The model under review builds one solid part; all positions refer to its coordinate system, in mm. Face numbers are marked on the shaded views. A direction names the side the tool comes from. Coordinates: 2 decimals unless noted, no trailing zeros. Write each loop counter-clockwise with the first axis right and the second up, starting at its lowest first coordinate (ties: lowest second). Pieces come first, ordered by that corner, then holes. Notation, with made-up numbers: (-15.75, 17) - (38.25, 17) arc R30 cw to (38.25, 51) - close; hole circle Ø7 at (50.5, 28.25). An arc over 180 degrees is marked (long way). Return JSON: item names as keys, results as strings. Group by question number.
(1) We need section A-A on z = -1. Give the number of separate pieces and of enclosed holes in the cut face, then the cut area to 3 significant figures.
(2) We need section C-C on z = 7. State the section outline as (x, y) points, then the cut area to 3 significant figures.
(3) Draft analysis for pull direction Y (two halves, no side actions). For the marked faces 1, 2, 3 and 4, state which applies: released by +Y, released by -Y, zero draft, split by the parting line, or undercut.
(4) To check wall thickness, follow L1, parallel to X at y = -2.75, z = 7; L2, parallel to Z at x = 0, y = -2.5; L3, parallel to Z at x = 0, y = -2. State the ranges of each line that lie inside material, in increasing order. Write a range as from..to.
(5) We need section B-B on x = 0. State the section outline as (y, z) points.
(6) We need section D-D on y = 0.5. State the section outline as (x, z) points.
(7) Tool access review of the marked faces 5, 6, 7 and 8: name each direction out of +Z, -Z, +X, -X, +Y, -Y from which nothing blocks a thin tool from reaching the whole face with its end or side.
(8) For pin 1 Ø0.9 at (x, z) = (4.5, -1) entering from +Y; pin 2 Ø3.5 at (x, y) = (-1.5, 4) entering from +Z; pin 3 Ø0.9 at (y, z) = (-4.5, -0.5) entering from -X, all flat-tipped, find the tip position at first contact; note any pin that passes through.
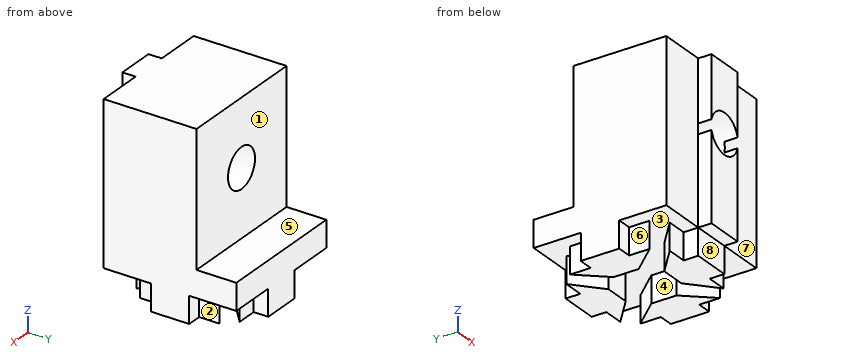
```python
from build123d import *

# Parameters (mm, degrees)
SKETCH1_W                         = 10
SKETCH1_H                         = 10
MAIN_DEPTH                        = 12
ANTIROTATIONSYSTEM_DEPTH          = 2
CIRPATTERN1_COUNT                 = 4
SKETCH3_W                         = 10
SKETCH3_H                         = 10
MAKERBEAMSQUAREHOLEFORSCREW_DEPTH = 3
SKETCH5_W                         = 2.9
SKETCH5_H                         = 12
MAKERBEAMRAIL_DEPTH               = 1
SKETCH4_R                         = 1.5
VERTICALMAKERBEAMHOLE_DEPTH       = 9


with BuildPart() as part:
    # Sketch1 → Main (new body)
    with BuildSketch(Plane.XY):
        Rectangle(SKETCH1_W, SKETCH1_H)
    extrude(amount=MAIN_DEPTH)

    # Sketch2 → AntiRotationSystem (add)
    with BuildSketch(Plane(origin=(0, 0, 0), x_dir=(-1, 0, 0), z_dir=(0, 0, -1))):
        Polygon((-5, 1.45), (-3.9, 1.45), (-3.9, 3), (-2.1, 0.95), (-2.1, -0.95), (-3.9, -3), (-3.9, -1.45), (-5, -1.45), align=None)
    antirotationsystem = extrude(amount=ANTIROTATIONSYSTEM_DEPTH)

    # CirPattern1: AntiRotationSystem ×4 about axis
    cirpattern1_axis = Axis((0, 0, 0), (0, 0, 1))
    for i in range(1, CIRPATTERN1_COUNT):
        add(antirotationsystem.rotate(cirpattern1_axis, i * 360 / CIRPATTERN1_COUNT))

    # Sketch3 → MakerBeamSquareHoleForScrew (cut)
    with BuildSketch(Plane(origin=(0, 5, 0), x_dir=(1, 0, 0), z_dir=(0, 1, 0))):
        with Locations((0, -7)):
            Rectangle(SKETCH3_W, SKETCH3_H)
    extrude(amount=-MAKERBEAMSQUAREHOLEFORSCREW_DEPTH, mode=Mode.SUBTRACT)

    # Sketch5 → MakerBeamRail (add)
    with BuildSketch(Plane(origin=(0, -5, 0), x_dir=(-1, 0, 0), z_dir=(0, -1, 0))):
        with Locations((0, -6)):
            Rectangle(SKETCH5_W, SKETCH5_H)
    extrude(amount=MAKERBEAMRAIL_DEPTH)

    # Sketch4 → VerticalMakerBeamHole (cut, through all)
    with BuildSketch(Plane(origin=(0, 2, 0), x_dir=(1, 0, 0), z_dir=(0, 1, 0))):
        with Locations((0, -7)):
            Circle(SKETCH4_R)
    extrude(amount=-VERTICALMAKERBEAMHOLE_DEPTH, mode=Mode.SUBTRACT)


solid = part.part
```
Ans:
{
 "1": {"separate pieces": "4", "enclosed holes": "0", "area": "41.2 mm²"},
 "2": {"outline": "(-5, -5) - (-1.5, -5) - (-1.5, 2) - (-5, 2) - close; (1.5, -5) - (5, -5) - (5, 2) - (1.5, 2) - close", "area": "49.0 mm²"},
 "3": {"face 1": "released by +Y", "face 2": "zero draft", "face 3": "undercut", "face 4": "undercut"},
 "4": {"L1": "-5..-1.5, 1.5..5", "L2": "-2..5.5, 8.5..12", "L3": "0..5.5, 8.5..12"},
 "5": {"outline": "(-6, 0) - (-5, 0) - (-5, -2) - (-2.1, -2) - (-2.1, 0) - (2.1, 0) - (2.1, -2) - (5, -2) - (5, 2) - (2, 2) - (2, 5.5) - (-6, 5.5) - close; (-6, 8.5) - (2, 8.5) - (2, 12) - (-6, 12) - close"},
 "6": {"outline": "(-5, -2) - (-2.1, -2) - (-2.1, 0) - (2.1, 0) - (2.1, -2) - (5, -2) - (5, 12) - (-5, 12) - close; hole circle Ø3 at (0, 7)"},
 "7": {"face 5": "+Z, +X, -X, +Y", "face 6": "-Z, -X, -Y", "face 7": "+Z, -Z, +X, -Y", "face 8": "-Z, +X, -X, -Y"},
 "8": {"pin 1": "y = 1.45", "pin 2": "z = 2", "pin 3": "x = -1.45"}
}
